```python
from build123d import *

# Parameters (mm, degrees)
IZIM1_W               = 152
IZIM1_H               = 12.405405405
IZIM2_R               = 4
KES_EKSTR_ZYON1_DEPTH = 21
KES_EKSTR_ZYON2_START = -21
KES_EKSTR_ZYON2_DEPTH = 21


with BuildPart() as part:
    # Çizim1 → Döndür1 (revolve)
    with BuildSketch(Plane(origin=(0, 0, 0), x_dir=(-1, 0, 0), z_dir=(0, 0, -1)), mode=Mode.PRIVATE) as d_nd_r1_sk:
        with Locations((-77, 6.202702703)):
            Rectangle(IZIM1_W, IZIM1_H)
    revolve(d_nd_r1_sk.sketch.rotate(Axis((153, 0, 0), (-1, 0, 0)), 270), axis=Axis((153, 0, 0), (-1, 0, 0)))

    # Çizim2 → Kes-Ekstrüzyon1 (cut)
    with BuildSketch(Plane(origin=(153, 0, 0), x_dir=(0, 0, -1), z_dir=(1, 0, 0))):
        Circle(IZIM2_R)
    extrude(amount=-KES_EKSTR_ZYON1_DEPTH, mode=Mode.SUBTRACT)

    # Çizim3 → Kes-Ekstrüzyon2 (cut)
    with BuildSketch(Plane.ZY.offset(-1).offset(KES_EKSTR_ZYON2_START)):
        with BuildLine():
            ThreePointArc((1.5, -3.708099244), (0, 4), (-1.5, -3.708099244))
            ThreePointArc((-1.5, -3.708099244), (0, -4), (1.5, -3.708099244))
        make_face()
    extrude(amount=KES_EKSTR_ZYON2_DEPTH, mode=Mode.SUBTRACT)


solid = part.part
```
Geometry: final body of the model. Coordinates: model frame, mm. A direction names the side the tool comes from. Give positions to 0.01 mm unless a question says otherwise; leave off trailing zeros. Write each loop counter-clockwise with the first axis right and the second up, starting at its lowest first coordinate (ties: lowest second). Pieces come first, ordered by that corner, then holes.
1. Section query C-C, the plane x = 135. Return loops of the section in (y, z).
2. Line query: probe 1 along Y at (x, z) = (7, 0); probe 2 along Y at (x, z) = (29, -0.25); probe 3 along X at (y, z) = (0.75, -3). Output: solid intervals per line, ascending.
3. Reachability of faces 1 (the flat face through (153, 3, 3)), 2 (the cylindrical face through (142.647, -3.905, 0.867)), 3 (the flat face through (22, 0, 0)) from +Z, -Z, +X, -X, +Y, -Y: full face, straight path, thin tool, end or side. Return the list, or none.
4. Section query D-D, the plane x = 108. Return loops of the section in (y, z).
5. Draft query along Z for faces 4 (the cylindrical face through (75.94, 3.73, 11.83)), 5 (the flat face through (132, 0, 0)), 6 (the flat face through (1, 3, 3)). Return one class per face: released by +Z, released by -Z, zero draft, split by the parting line, or undercut.
6. Pin query (flat end, axial travel): P1, Ø4, axis at y = 0, z = -1, coming from the +X side; P2, Ø6.5, axis at y = 0.5, z = 0, coming from the -X side; P3, Ø1, axis at x = 126.5, z = -1.5, coming from the -Y side. Return the tip coordinate at first contact, or that it passes through.
7. Section query A-A, the plane y = 0. Return loops of the section in (x, z).
Computed:
1. outline: circle Ø24.81 at (0, 0); hole circle Ø8 at (0, 0)
2. probe 1: y = -12.41 to -4, 4 to 12.41
2. probe 2: y = -12.4 to 12.4
2. probe 3: x = 22 to 132
3. face 1: +Z, -Z, +X, +Y, -Y
3. face 2: +X
3. face 3: -X
4. outline: circle Ø24.81 at (0, 0)
5. face 4: split by the parting line
5. face 5: undercut
5. face 6: zero draft
6. P1: stops at x = 132
6. P2: stops at x = 22
6. P3: stops at y = -12.37
7. outline: (1, -12.41) - (153, -12.41) - (153, -4) - (132, -4) - (132, 4) - (153, 4) - (153, 12.41) - (1, 12.41) - (1, 4) - (22, 4) - (22, -4) - (1, -4) - close
